```python
from build123d import *

# Parameters (mm, degrees)
F0_R     = 150
F0_R_2   = 125
F1_DEPTH = 120
F2_R     = 5


with BuildPart() as f1:
    # F0 (on Right) → F1 (new body)
    with BuildSketch(Plane.YZ):
        Circle(F0_R)
        Circle(F0_R_2, mode=Mode.SUBTRACT)
    extrude(amount=F1_DEPTH)

    # F2
    f2_edges = [f1.edges().sort_by_distance(p)[0] for p in [
        (120, -125, 0),
        (120, -150, 0),
        (0, -150, 0),
        (0, -125, 0),
    ]]
    fillet(f2_edges, radius=F2_R)


solid = f1.part
```
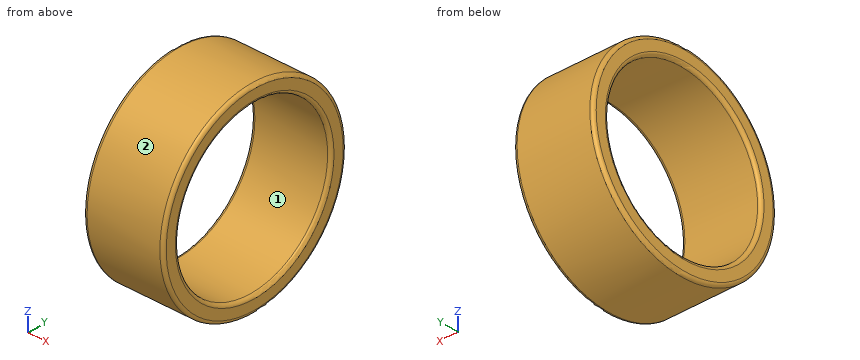
CAD build for the part. Positions are in the model's coordinates, mm. Face numbers are marked on the shaded views. Give positions to 0.01 mm unless a question says otherwise; leave off trailing zeros. Loops run counter-clockwise (first coordinate to the right, second up) from the corner with the lowest first, then second, coordinate; pieces in that order, holes last. Notation, with made-up numbers: (48, 82) -> (103, 82) arc R14 ccw to (103, 107) -> close; hole circle Ø5 at (-19.5, 85). An arc over 180 degrees is marked (long way). Use a Markdown table: item, result.
1. Mould opens along Z. For the marked faces 1 and 2 say: pulls with the +Z half, pulls with the -Z half, needs draft (parallel to the pull), parting line crosses it, or undercut.
Check result:
| item | result |
|---|---|
| face 1 | undercut |
| face 2 | parting line crosses it |
2. Flat gauge pins, fed straight in: pin 1 (12 mm diameter, centred on x = 22, y = -107, fed in from -Z); pin 2 (4 mm diameter, centred on x = 44, z = 48, fed in from -Y); pin 3 (6 mm diameter, centred on x = 75.5, z = -42, fed in from -Y). Where does each tip first touch, or does it go through?
Check result:
| item | result |
|---|---|
| pin 1 | stops at z = -110.9 |
| pin 2 | stops at y = -142.77 |
| pin 3 | stops at y = -144.84 |
3. Slice it at A-A (z = 0). List the corners of the cut face in (x, y).
Check result:
| item | result |
|---|---|
| outline | (0, -145) arc R5 ccw to (5, -150) -> (115, -150) arc R5 ccw to (120, -145) -> (120, -130) arc R5 ccw to (115, -125) -> (5, -125) arc R5 ccw to (0, -130) -> close; (0, 130) arc R5 ccw to (5, 125) -> (115, 125) arc R5 ccw to (120, 130) -> (120, 145) arc R5 ccw to (115, 150) -> (5, 150) arc R5 ccw to (0, 145) -> close |
4. Slice it at C-C (x = 70). List the corners of the cut face in (y, z), plus the area to 3 significant figures.
Check result:
| item | result |
|---|---|
| outline | circle Ø300 at (0, 0); hole circle Ø250 at (0, 0) |
| area | 21,600 mm^2 |
5. Wall check: L1, parallel to Z at x = 54.5, y = 0; L2, parallel to Y at x = 56, z = 70 (3 decimals); L3, parallel to Z at x = 8, y = 59. Give the ranges that are in metal, low to high. Write a range as [from, to].
Check result:
| item | result |
|---|---|
| L1 | z = [-150, -125], [125, 150] |
| L2 | y = [-132.665, -103.562], [103.562, 132.665] |
| L3 | z = [-137.91, -110.2], [110.2, 137.91] |
